Work out the finished part from the listing and answer in its coordinate system (mm). Face numbers are marked on the shaded views. A direction names the side the tool comes from. Coordinates: 2 decimals unless noted, no trailing zeros. Order: outer loops, then holes, each group sorted by start corner. A loop starts at its lowest first (then second) coordinate and runs counter-clockwise, first axis right, second up. Notation, with made-up numbers: (86.25, 55) - (143.25, 55) arc R37 ccw to (143.25, 94) - close; hole circle Ø8 at (30.25, 9). An arc over 180 degrees is marked (long way). Use CSV: the item, a comma, the result in double quotes. Start each with the question number.
from build123d import *

# Parameters (mm, degrees)
F0_W     = 88.9
F0_H     = 127
F0_W_2   = 69.85
F0_H_2   = 101.6
F1_DEPTH = 6.35
F2_R     = 3.175
F3_DEPTH = 6.35


with BuildPart() as f1:
    # F0 (on Top) → F1 (new body)
    with BuildSketch(Plane.XY):
        with Locations((-20.780801, 12.657491)):
            Rectangle(F0_W, F0_H)
        with Locations((-20.780801, 15.832491)):
            Rectangle(F0_W_2, F0_H_2, mode=Mode.SUBTRACT)
    extrude(amount=F1_DEPTH)

    # F2 (on face) → F3 (join)
    with BuildSketch(Plane.XY.offset(6.35)):
        with Locations((-58.880801, 69.807491)):
            Circle(F2_R)
        with Locations((-58.880801, -31.792509)):
            Circle(F2_R)
        with Locations((17.319199, 69.807491)):
            Circle(F2_R)
        with Locations((17.319199, -31.792509)):
            Circle(F2_R)
    extrude(amount=F3_DEPTH)


solid = f1.part
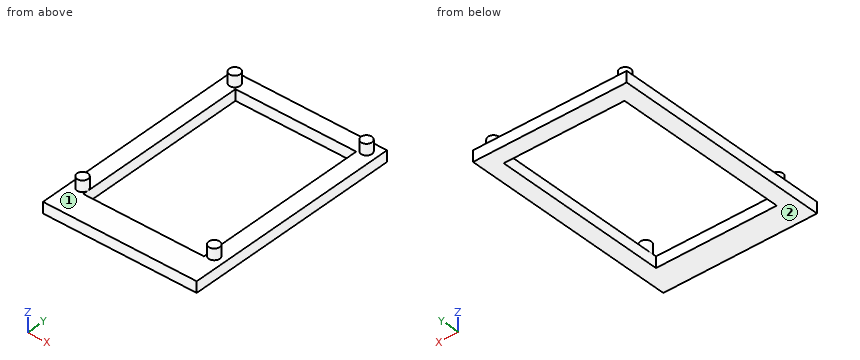
1) The part is cut by section D-D on y = -42.5. Determine the outline of the cut face in (x, z), plus the area to 3 significant figures.
2) The part is cut by section B-B on x = -46.5. Determine the outline of the cut face in (y, z).
3) Straight lines are drawn through the part: line 1 (X direction, y = 14, z = 2.5); line 2 (Y direction, x = -39, z = 5.25); line 3 (Z direction, x = -39.5, y = 67). For each, find the intervals that lie inside material, in ascending order. Write a range as [from, to].
4) The part is cut by section A-A on y = -25.5. Determine the outline of the cut face in (x, z), plus the area to 3 significant figures.
5) A flat-ended cylindrical pin translates along its axis: P1, Ø2, axis at x = -54.5, z = 11, coming from the +Y side. Find the tip coordinate at first contact, or state that the pin passes through.
6) For the marked faces 1 and 2, determine the directions among +Z, -Z, +X, -X, +Y, -Y from which every point of the face is accessible in a straight line to the end or side of a thin tool.
7) The part is cut by section C-C on z = 2.75. Determine the outline of the cut face in (x, y), plus the area to 3 significant figures.
Answer key:
1,outline,"(-65.23, 0) - (23.67, 0) - (23.67, 6.35) - (-65.23, 6.35) - close"
1,area,"565 mm^2"
2,outline,"(-50.84, 0) - (-34.97, 0) - (-34.97, 6.35) - (-50.84, 6.35) - close; (66.63, 0) - (76.16, 0) - (76.16, 6.35) - (66.63, 6.35) - close"
3,line 1,"[-65.23, -55.71], [14.14, 23.67]"
3,line 2,"[-50.84, -34.97], [66.63, 76.16]"
3,line 3,"[0, 6.35]"
4,outline,"(-65.23, 0) - (-55.71, 0) - (-55.71, 6.35) - (-65.23, 6.35) - close; (14.14, 0) - (23.67, 0) - (23.67, 6.35) - (14.14, 6.35) - close"
4,area,"121 mm^2"
5,P1,"through"
6,face 1,"+Z"
6,face 2,"-Z, +X, -X, +Y, -Y"
7,outline,"(-65.23, -50.84) - (23.67, -50.84) - (23.67, 76.16) - (-65.23, 76.16) - close; hole (-55.71, -34.97) - (14.14, -34.97) - (14.14, 66.63) - (-55.71, 66.63) - close"
7,area,"4,190 mm^2"
